Could you check a few things on this model? Use its own coordinates, in mm. Give positions to 0.01 mm unless a question says otherwise; leave off trailing zeros. Write each loop counter-clockwise with the first axis right and the second up, starting at its lowest first coordinate (ties: lowest second). Pieces come first, ordered by that corner, then holes. Notation, with made-up numbers: M 38,36 L 95,36 A18 ccw 95,59 Z; hole C 0,5 d5. An arc over 180 degrees is marked long. One line per item, written item: value.
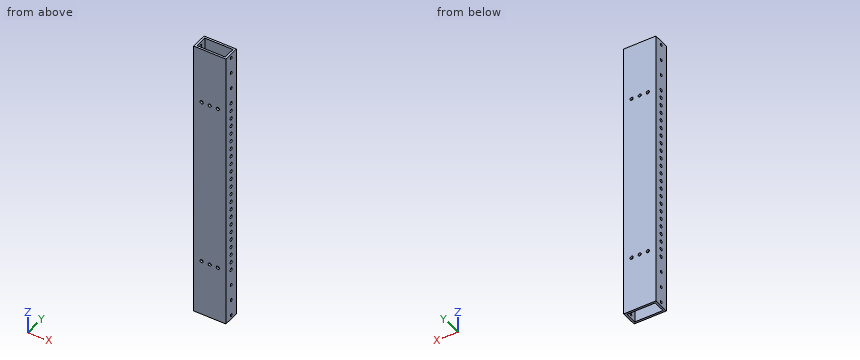
```python
from build123d import *

# Parameters (mm, degrees)
SKETCH1_W           = 50.8
SKETCH1_H           = 25.4
SKETCH1_W_2         = 44.45
SKETCH1_H_2         = 19.05
BOSS_EXTRUDE1_DEPTH = 222.25
SKETCH3_R           = 2.15265
SKETCH3_R_2         = 2.159
CUT_EXTRUDE2_DEPTH  = 51.8
SKETCH4_R           = 2.4892
CUT_EXTRUDE3_DEPTH  = 51.8
SKETCH5_R           = 2.4892
CUT_EXTRUDE4_DEPTH  = 26.4


with BuildPart() as part:
    # Sketch1 → Boss-Extrude1 (new body, symmetric)
    with BuildSketch(Plane.XY):
        Rectangle(SKETCH1_W, SKETCH1_H)
        Rectangle(SKETCH1_W_2, SKETCH1_H_2, mode=Mode.SUBTRACT)
    extrude(amount=BOSS_EXTRUDE1_DEPTH, both=True)

    # Sketch3 → Cut-Extrude2 (cut, through all)
    with BuildSketch(Plane(origin=(25.4, 0, 0), x_dir=(0, 0, -1), z_dir=(1, 0, 0))):
        with Locations((-215.9, 0)):
            Circle(SKETCH3_R)
        with Locations((-190.5, 0)):
            Circle(SKETCH3_R)
        with Locations((-165.1, 0)):
            Circle(SKETCH3_R)
        with Locations((215.9, 0)):
            Circle(SKETCH3_R_2)
        with Locations((190.5, 0)):
            Circle(SKETCH3_R_2)
        with Locations((165.1, 0)):
            Circle(SKETCH3_R_2)
    extrude(amount=-CUT_EXTRUDE2_DEPTH, mode=Mode.SUBTRACT)

    # Sketch4 → Cut-Extrude3 (cut, through all)
    with BuildSketch(Plane(origin=(25.4, 0, 0), x_dir=(0, 0, -1), z_dir=(1, 0, 0))):
        with Locations((-139.7, 0)):
            Circle(SKETCH4_R)
        with Locations((-127, 0)):
            Circle(SKETCH4_R)
        with Locations((-114.3, 0)):
            Circle(SKETCH4_R)
        with Locations((-101.6, 0)):
            Circle(SKETCH4_R)
        with Locations((-88.9, 0)):
            Circle(SKETCH4_R)
        with Locations((-76.2, 0)):
            Circle(SKETCH4_R)
        with Locations((-63.5, 0)):
            Circle(SKETCH4_R)
        with Locations((-50.8, 0)):
            Circle(SKETCH4_R)
        with Locations((-38.1, 0)):
            Circle(SKETCH4_R)
        with Locations((-25.4, 0)):
            Circle(SKETCH4_R)
        with Locations((-12.7, 0)):
            Circle(SKETCH4_R)
        Circle(SKETCH4_R)
        with Locations((12.7, 0)):
            Circle(SKETCH4_R)
        with Locations((25.4, 0)):
            Circle(SKETCH4_R)
        with Locations((38.1, 0)):
            Circle(SKETCH4_R)
        with Locations((50.8, 0)):
            Circle(SKETCH4_R)
        with Locations((63.5, 0)):
            Circle(SKETCH4_R)
        with Locations((76.2, 0)):
            Circle(SKETCH4_R)
        with Locations((88.9, 0)):
            Circle(SKETCH4_R)
        with Locations((101.6, 0)):
            Circle(SKETCH4_R)
        with Locations((114.3, 0)):
            Circle(SKETCH4_R)
        with Locations((127, 0)):
            Circle(SKETCH4_R)
        with Locations((139.7, 0)):
            Circle(SKETCH4_R)
    extrude(amount=-CUT_EXTRUDE3_DEPTH, mode=Mode.SUBTRACT)

    # Sketch5 → Cut-Extrude4 (cut, through all)
    with BuildSketch(Plane.XZ.offset(12.7)):
        with Locations((-12.7, 133.35)):
            Circle(SKETCH5_R)
        with Locations((0, 133.35)):
            Circle(SKETCH5_R)
        with Locations((12.7, 133.35)):
            Circle(SKETCH5_R)
        with Locations((12.7, -133.35)):
            Circle(SKETCH5_R)
        with Locations((0, -133.35)):
            Circle(SKETCH5_R)
        with Locations((-12.7, -133.35)):
            Circle(SKETCH5_R)
    extrude(amount=-CUT_EXTRUDE4_DEPTH, mode=Mode.SUBTRACT)


solid = part.part
```
1) I'm going to push a flat-ended pin straight in: pin 1 (4.5 mm diameter, centred on y = 0, z = 101.6, fed in from -X). Where does the tip first touch, or does it pass through?
Outcome:
pin 1: passes through
2) Please list where these lines run through material, in increasing order: L1, parallel to X at y = 10.75, z = 133.35; L2, parallel to X at y = 8, z = 56.5 (3 decimals); L3, parallel to Y at x = 0.5, z = 122.5 (3 decimals). Write a range as from..to.
Outcome:
L1: x = -25.4..-15.19, -10.21..-2.49, 2.49..10.21, 15.19..25.4
L2: x = -25.4..-22.225, 22.225..25.4
L3: y = -12.7..-9.525, 9.525..12.7
3) If we section it at A-A, the plane z = 158: Write out the boundary of the cut face in (x, y) (3 decimals), then the cut area to 3 significant figures.
Outcome:
outline: M -25.4,-12.7 L 25.4,-12.7 L 25.4,12.7 L -25.4,12.7 Z; hole M -22.225,-9.525 L 22.225,-9.525 L 22.225,9.525 L -22.225,9.525 Z
area: 444 mm^2
